Input: part model. Units: mm. Frame: model coordinates. A direction names the side the tool comes from. Coordinates: 2 decimals unless noted, no trailing zeros. Loops run counter-clockwise (first coordinate to the right, second up) from the corner with the lowest first, then second, coordinate; pieces in that order, holes last. Notation, with made-up numbers: (1, 1.25) - (5, 1.25) arc R21 ccw to (5, 29.25) - close; hole circle Ø9 at (55, 48.25). An arc over 180 degrees is marked (long way). Write item = value, one per line. Start each with the question number.
from build123d import *

# Parameters (mm, degrees)
BOSS_EXTRUDE1_DEPTH = 3.556


with BuildPart() as part:
    # Sketch1 → Boss-Extrude1 (new body)
    with BuildSketch(Plane.XY):
        Polygon((27.81, -3.556), (27.81, 3.556), (22.81, 3.556), (22.81, 2.28), (20.81, 2.28), (20.81, 3.556), (16.13, 3.556), (16.13, 1.795), (14.13, 1.795), (14.13, 3.556), (8.63, 3.556), (8.63, 1.695), (6.63, 1.695), (6.63, 3.556), (1, 3.556), (1, 1.68), (-1, 1.68), (-1, 3.556), (-6.63, 3.556), (-6.63, 1.695), (-8.63, 1.695), (-8.63, 3.556), (-14.13, 3.556), (-14.13, 1.795), (-16.13, 1.795), (-16.13, 3.556), (-20.81, 3.556), (-20.81, 2.28), (-22.81, 2.28), (-22.81, 3.556), (-27.81, 3.556), (-27.81, -3.556), (-22.81, -3.556), (-22.81, -2.28), (-20.81, -2.28), (-20.81, -3.556), (-16.13, -3.556), (-16.13, -1.795), (-14.13, -1.795), (-14.13, -3.556), (-8.63, -3.556), (-8.63, -1.695), (-6.63, -1.695), (-6.63, -3.556), (-1, -3.556), (-1, -1.68), (1, -1.68), (1, -3.556), (6.63, -3.556), (6.63, -1.695), (8.63, -1.695), (8.63, -3.556), (14.13, -3.556), (14.13, -1.795), (16.13, -1.795), (16.13, -3.556), (20.81, -3.556), (20.81, -2.28), (22.81, -2.28), (22.81, -3.556), align=None)
    extrude(amount=BOSS_EXTRUDE1_DEPTH)


solid = part.part
Item 1: Cut plane C-C on x = -22. Return loops of the section in (y, z).
Item 2: Access query for faces 5 (the flat face through (0, 0, 0)), 6 (the flat face through (-8, -1.695, 2)), 7 (the flat face through (0, 1.68, 2)). Directions: +Z, -Z, +X, -X, +Y, -Y. A direction counts if a zero-diameter tool reaches every point of the face in a straight line with its end or side. Return the directions, or none.
Item 3: Cut plane B-B on x = 8. Return loops of the section in (y, z) (3 decimals), plus the area to 3 significant figures.
Item 4: Ray query, line 1 (X direction, y = -2.25, z = 1.25); line 2 (Y direction, x = -15.5, z = 1.9) (3 decimals); line 3 (Y direction, x = 21, z = 0.8). Return the intervals inside material, ascending.
Item 5: Pin query (flat end, axial travel): pin 1 (0.6 mm diameter, centred on x = -8, z = 1.5, fed in from +Y) (3 decimals); pin 2 (0.6 mm diameter, centred on x = -14.5, z = 1, fed in from -Y) (3 decimals). Return the tip coordinate at first contact, or that it passes through.
Item 6: Pull-direction query (X, two-part tool) for faces 1 (the flat face through (20.81, 3, 2)), 2 (the flat face through (11, -3.556, 2)), 3 (the flat face through (8, -1.695, 2)), 4 (the flat face through (27.81, 0, 2)); classes: pulls with the +X half, pulls with the -X half, needs draft (parallel to the pull), parting line crosses it, or undercut.
Item 7: Cut plane A-A on y = 2.75. State how many separate pieces and enclosed holes the cut face has, plus the area to 3 significant figures.
Recorded:
q1.outline = (-2.28, 0) - (2.28, 0) - (2.28, 3.56) - (-2.28, 3.56) - close
q2.face_5 = -Z, +X, -X, +Y, -Y
q2.face_6 = +Z, -Z, -Y
q2.face_7 = +Z, -Z, +Y
q3.outline = (-1.695, 0) - (1.695, 0) - (1.695, 3.556) - (-1.695, 3.556) - close
q3.area = 12.1 mm²
q4.line_1 = -27.81 to -16.13, -14.13 to -8.63, -6.63 to -1, 1 to 6.63, 8.63 to 14.13, 16.13 to 27.81
q4.line_2 = -1.795 to 1.795
q4.line_3 = -2.28 to 2.28
q5.pin_1 = 1.695
q5.pin_2 = -1.795
q6.face_1 = undercut
q6.face_2 = needs draft
q6.face_3 = undercut
q6.face_4 = pulls with the +X half
q7.separate_pieces = 8
q7.enclosed_holes = 0
q7.area = 148 mm²
